For this review, use the dimensioned drawing (mm, ordinates from the lowest corner) and the shaded views. Coordinates: 2 decimals unless noted, no trailing zeros. Order: outer loops, then holes, each group sorted by start corner. A loop starts at its lowest first (then second) coordinate and runs counter-clockwise, first axis right, second up. Notation, with made-up numbers: M 86,16.25 L 144,16.25 A21 ccw 144,28.25 Z; hole C 79.25,81.5 d1. An arc over 180 degrees is marked long. Answer in a Markdown table with one row per item.
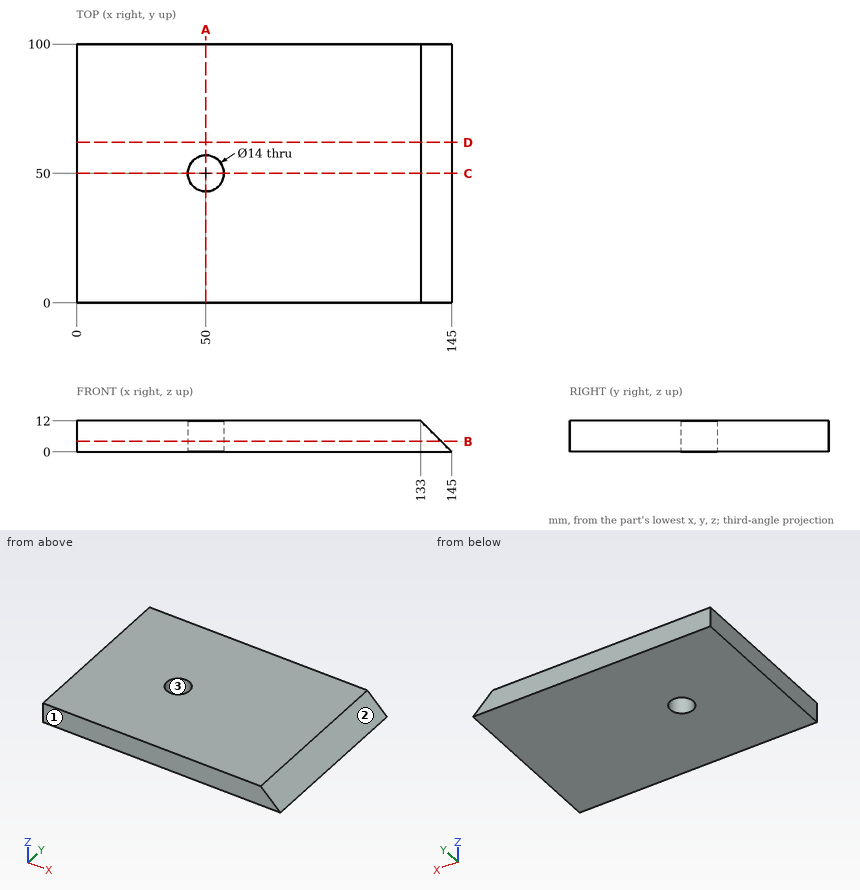
(1) Add section D-D, the plane y = 62. Give the boundary of the cut face in (x, z).
Return value:
| item | result |
|---|---|
| outline | M 0,0 L 145,0 L 133,12 L 0,12 Z |
(2) Add section A-A, the plane x = 50. Give the boundary of the cut face in (y, z), and give its area (3 significant figures).
Return value:
| item | result |
|---|---|
| outline | M 0,0 L 43,0 L 43,12 L 0,12 Z; M 57,0 L 100,0 L 100,12 L 57,12 Z |
| area | 1,030 mm2 |
(3) For line 1 along Y through (x, z) = (50, 2.5); line 2 along X through (y, z) = (52.5, 10.5); line 3 along X through (y, z) = (50, 7), list the stretches that pass through material, from the lowest coordinate up. Write a range as from..to.
Return value:
| item | result |
|---|---|
| line 1 | y = 0..43, 57..100 |
| line 2 | x = 0..43.46, 56.54..134.5 |
| line 3 | x = 0..43, 57..138 |
(4) Add section C-C, the plane y = 50. Give the boundary of the cut face in (x, z), and give its area (3 significant figures).
Return value:
| item | result |
|---|---|
| outline | M 0,0 L 43,0 L 43,12 L 0,12 Z; M 57,0 L 145,0 L 133,12 L 57,12 Z |
| area | 1,500 mm2 |
(5) Add section B-B, the plane z = 4. Give the boundary of the cut face in (x, y), and give its area (3 significant figures).
Return value:
| item | result |
|---|---|
| outline | M 0,0 L 141,0 L 141,100 L 0,100 Z; hole C 50,50 d14 |
| area | 13,900 mm2 |
(6) Draft analysis for pull direction Y (two halves, no side actions). For the marked faces 1, 2 and 3, state which applies: pulls with the +Y half, pulls with the -Y half, needs draft (parallel to the pull), parting line crosses it, or undercut.
Return value:
| item | result |
|---|---|
| face 1 | pulls with the -Y half |
| face 2 | needs draft |
| face 3 | undercut |
(7) Insertion check: pin 1 Ø2 at (x, z) = (34.5, 6.5) entering from -Y; pin 2 Ø2 at (y, z) = (32, 3.5) entering from +X. Each pin has a flat end and moves straight along its axis. Give the tip position at first contact, or say it passes through.
Return value:
| item | result |
|---|---|
| pin 1 | stops at y = 0 |
| pin 2 | stops at x = 142.5 |
